```python
from build123d import *

# Parameters (mm, degrees)
SKETCH_2_R      = 2.5
SKETCH_2_R_2    = 6
EXTRUDE_1_DEPTH = 5


with BuildPart() as part:
    # 草图2 → 凸台-拉伸1 (new body)
    with BuildSketch(Plane(origin=(0, 0, 0), x_dir=(1, 0, 0), z_dir=(0, 1, 0))):
        with BuildLine():
            Line((25.631960973, 178.867513459), (-49.971960973, 178.867513459))
            ThreePointArc((-49.971960973, 178.867513459), (-57.705382386, 175.207402516), (-59.77776773, 166.906352108))
            Line((-59.77776773, 166.906352108), (-41.587420271, 75.954614813))
            ThreePointArc((-41.587420271, 75.954614813), (-12.17, 51.838098867), (17.247420271, 75.954614813))
            Line((17.247420271, 75.954614813), (35.43776773, 166.906352108))
            ThreePointArc((35.43776773, 166.906352108), (33.365382386, 175.207402516), (25.631960973, 178.867513459))
        make_face()
        with Locations(Location((-30.17, 78.867513459, 0), (0, 0, 270))):
            Circle(SKETCH_2_R, mode=Mode.SUBTRACT)
        with Locations(Location((5.83, 78.867513459, 0), (0, 0, 90))):
            Circle(SKETCH_2_R, mode=Mode.SUBTRACT)
        with Locations(Location((-50, 168.867513459, 0), (0, 0, 270))):
            Circle(SKETCH_2_R, mode=Mode.SUBTRACT)
        with Locations(Location((25.66, 168.867513459, 0), (0, 0, 90))):
            Circle(SKETCH_2_R, mode=Mode.SUBTRACT)
        with Locations(Location((-12.17, 78.867513459, 0), (0, 0, 270))):
            Circle(SKETCH_2_R_2, mode=Mode.SUBTRACT)
    extrude(amount=EXTRUDE_1_DEPTH)


solid = part.part
```
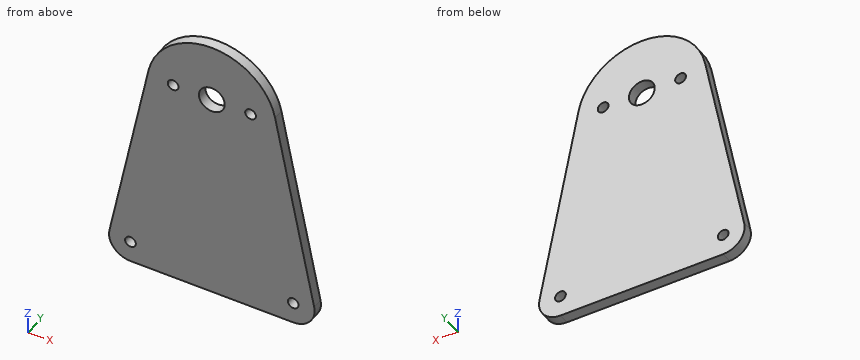
Here's how the part is built. I have some questions about the finished solid (model axes, mm). Coordinates: 2 decimals unless noted, no trailing zeros. Order: outer loops, then holes, each group sorted by start corner. A loop starts at its lowest first (then second) coordinate and runs counter-clockwise, first axis right, second up. Notation, with made-up numbers: M -24,71.5 L -8,71.5 A22 ccw -8,104.5 Z; hole C -26.75,-5 d2. An arc over 180 degrees is marked long. Answer as a JSON object with one key per item and string values. Group by question number.
(1) For pin 1 (6.5 mm diameter, centred on x = 5.83, z = -78.87, fed in from -Y), with a flat end and sliding along its axis, tell me the tip position at first contact or that it passes through.
(2) Suppose I cut it at A-A, the plane x = -12.17. Please give me the cut outline in (y, z), then the cut area to 3 significant figures.
(3) Suppose I cut it at D-D, the plane x = 5.83. Please give me the cut outline in (y, z), then the cut area to 3 significant figures.
(4) Suppose I cut it at B-B, the plane y = 1.8. Please give me the cut outline in (x, z), then the cut area to 3 significant figures.
(5) Suppose I cut it at C-C, the plane z = -79.5. Please give me the cut outline in (x, y).
(6) I need wall thicknesses on probe 1 along X at (y, z) = (0.5, -168); probe 2 along X at (y, z) = (2.9, -79); probe 3 along X at (y, z) = (3.85, -108). Which ranges of each line are inside material? Lowest first, please.
Values found:
{
 "1": {"pin 1": "stops at y = 0"},
 "2": {"outline": "M 0,-178.87 L 5,-178.87 L 5,-84.87 L 0,-84.87 Z; M 0,-72.87 L 5,-72.87 L 5,-51.84 L 0,-51.84 Z", "area": "575 mm^2"},
 "3": {"outline": "M 0,-178.87 L 5,-178.87 L 5,-81.37 L 0,-81.37 Z; M 0,-76.37 L 5,-76.37 L 5,-57.84 L 0,-57.84 Z", "area": "580 mm^2"},
 "4": {"outline": "M -59.78,-166.91 A10 ccw -49.97,-178.87 L 25.63,-178.87 A10 ccw 35.44,-166.91 L 17.25,-75.95 A30 ccw -41.59,-75.95 Z; hole C -50,-168.87 d5; hole C -30.17,-78.87 d5; hole C -12.17,-78.87 d12; hole C 5.83,-78.87 d5; hole C 25.66,-168.87 d5", "area": "8,980 mm^2"},
 "5": {"outline": "M -42.3,0 L -32.59,0 L -32.59,5 L -42.3,5 Z; M -27.75,0 L -18.14,0 L -18.14,5 L -27.75,5 Z; M -6.2,0 L 3.41,0 L 3.41,5 L -6.2,5 Z; M 8.25,0 L 17.96,0 L 17.96,5 L 8.25,5 Z"},
 "6": {"probe 1": "x = -59.93 to -52.34, -47.66 to 23.32, 28 to 35.59", "probe 2": "x = -42.2 to -32.67, -27.67 to -18.17, -6.17 to 3.33, 8.33 to 17.86", "probe 3": "x = -48 to 23.66"}
}
